For this review, take the finished solid that the model builds, in its own axes (mm). Face numbers are marked on the shaded views. A direction names the side the tool comes from. Coordinates: 2 decimals unless noted, no trailing zeros. Order: outer loops, then holes, each group sorted by start corner. A loop starts at its lowest first (then second) coordinate and runs counter-clockwise, first axis right, second up. Notation, with made-up numbers: (11.25, 24) -> (67.25, 24) arc R28 ccw to (67.25, 42) -> close; hole circle Ø1 at (5, 89.25). An arc over 180 degrees is marked (long way). Answer as a JSON object with one key per item and string values. Group by question number.
1) Add section C-C, the plane y = -20.5. Count the separate pieces of the cut face and the enclosed holes in it, then the cut area to 3 significant figures.
2) Add section B-B, the plane y = -36. Write out the cut boundary in (x, z).
3) Machinability: for the marked faces 1, 2, 3 and 4, which of the approach directions +Z, -Z, +X, -X, +Y, -Y give a long, thin tool a straight path to every point of the face, cutting with its end or side? Answer none if there is none.
4) For pin 1 (9 mm diameter, centred on y = -14, z = -31.5, fed in from -X); pin 2 (1 mm diameter, centred on y = -21, z = -8.5, fed in from +X); pin 3 (9 mm diameter, centred on y = -7.5, z = -28, fed in from +X); pin 4 (8 mm diameter, centred on x = 0.5, y = -35, fed in from +Z), all flat-tipped, find the tip position at first contact; note any pin that passes through.
5) Add section A-A, the plane z = 0. Write out the cut boundary in (x, y).
6) Add section D-D, the plane x = -16.5. Write out the cut boundary in (y, z), then the cut area to 3 significant figures.
7) Wall thickness on L1, parallel to X at y = -8, z = -29.5; L2, parallel to Z at x = 21.5, y = -3.5; L3, parallel to X at y = -27.5, z = -12.5: over which ranges is each line inside the solid? List them lowest first.
8) Draft analysis for pull direction X (two halves, no side actions). For the marked faces 5 and 6, state which applies: +X half, -X half, draft (parallel to the pull), parting line (faces both ways), or undercut.
from build123d import *

# Parameters (mm, degrees)
F0_W     = 86.6790302098
F0_H     = 110.9990477562
F0_R     = 4.1600175763
F0_R_2   = 4.0127427681
F1_DEPTH = 29.40571
F2_R     = 16.2901854198
F3_DEPTH = 25.4
F2_R_2   = 18.5490265687
F4_DEPTH = 30.0706941634
F6_R     = 15.7455659212
F7_DEPTH = 53.42441


with BuildPart() as f1:
    # F0 (on Front) → F1 (new body)
    with BuildSketch(Plane.XZ):
        with Locations((-5.9241037816, -20.7343772054)):
            Rectangle(F0_W, F0_H)
        with Locations((-28.4816268831, -32.2692543268)):
            Circle(F0_R, mode=Mode.SUBTRACT)
        with Locations((14.5424827933, -32.2692543268)):
            Circle(F0_R_2, mode=Mode.SUBTRACT)
        with BuildLine():
            add(Edge.make_bspline(
                [(-29.8793415714, -15.1079879142), (-29.0187247447, -16.080656118), (-29.0187247447, -17.7925521566)],
                knots=[0, 0, 0, 1, 1, 1], degree=2))
            add(Edge.make_bspline(
                [(-29.0187247447, -17.7925521566), (-29.0187247447, -19.4997793878), (-29.8824541096, -20.4778945335)],
                knots=[0, 0, 0, 1, 1, 1], degree=2))
            add(Edge.make_bspline(
                [(-29.8824541096, -20.4778945335), (-30.7461834745, -21.4560096792), (-32.2822211019, -21.4560096792)],
                knots=[0, 0, 0, 1, 1, 1], degree=2))
            add(Edge.make_bspline(
                [(-32.2822211019, -21.4560096792), (-33.8524966501, -21.4560096792), (-34.7061102657, -20.4950134939)],
                knots=[0, 0, 0, 1, 1, 1], degree=2))
            add(Edge.make_bspline(
                [(-34.7061102657, -20.4950134939), (-35.5597238813, -19.5340173086), (-35.5597238813, -17.7832145419)],
                knots=[0, 0, 0, 1, 1, 1], degree=2))
            add(Edge.make_bspline(
                [(-35.5597238813, -17.7832145419), (-35.5597238813, -16.0464181972), (-34.703775862, -15.0908689538)],
                knots=[0, 0, 0, 1, 1, 1], degree=2))
            add(Edge.make_bspline(
                [(-34.703775862, -15.0908689538), (-33.8478278427, -14.1353197105), (-32.2728834872, -14.1353197105)],
                knots=[0, 0, 0, 1, 1, 1], degree=2))
            add(Edge.make_bspline(
                [(-32.2728834872, -14.1353197105), (-30.739958398, -14.1353197105), (-29.8793415714, -15.1079879142)],
                knots=[0, 0, 0, 1, 1, 1], degree=2))
        make_face(mode=Mode.SUBTRACT)
        with BuildLine():
            Line((-23.1002332584, -21.3579647243), (-23.9079369348, -21.3579647243))
            Line((-23.9079369348, -21.3579647243), (-23.9079369348, -17.9092723411))
            add(Edge.make_bspline(
                [(-23.9079369348, -17.9092723411), (-23.9079369348, -17.2587518464), (-24.2044062034, -16.9373822719)],
                knots=[0, 0, 0, 1, 1, 1], degree=2))
            add(Edge.make_bspline(
                [(-24.2044062034, -16.9373822719), (-24.5008754719, -16.6160126973), (-25.1342770061, -16.6160126973)],
                knots=[0, 0, 0, 1, 1, 1], degree=2))
            add(Edge.make_bspline(
                [(-25.1342770061, -16.6160126973), (-25.9699935268, -16.6160126973), (-26.3590608083, -17.0681088784)],
                knots=[0, 0, 0, 1, 1, 1], degree=2))
            add(Edge.make_bspline(
                [(-26.3590608083, -17.0681088784), (-26.7481280898, -17.5202050596), (-26.7481280898, -18.5613491049)],
                knots=[0, 0, 0, 1, 1, 1], degree=2))
            Line((-26.7481280898, -18.5613491049), (-26.7481280898, -21.3579647243))
            Line((-26.7481280898, -21.3579647243), (-27.5558317662, -21.3579647243))
            Line((-27.5558317662, -21.3579647243), (-27.5558317662, -16.0277429677))
            Line((-27.5558317662, -16.0277429677), (-26.899086195, -16.0277429677))
            Line((-26.899086195, -16.0277429677), (-26.7683595885, -16.7576331878))
            Line((-26.7683595885, -16.7576331878), (-26.7294528603, -16.7576331878))
            add(Edge.make_bspline(
                [(-26.7294528603, -16.7576331878), (-26.4804498001, -16.3638970989), (-26.0330224264, -16.1467975558)],
                knots=[0, 0, 0, 1, 1, 1], degree=2))
            add(Edge.make_bspline(
                [(-26.0330224264, -16.1467975558), (-25.5855950527, -15.9296980128), (-25.0362320512, -15.9296980128)],
                knots=[0, 0, 0, 1, 1, 1], degree=2))
            add(Edge.make_bspline(
                [(-25.0362320512, -15.9296980128), (-24.0729014622, -15.9296980128), (-23.5865673603, -16.3942443469)],
                knots=[0, 0, 0, 1, 1, 1], degree=2))
            add(Edge.make_bspline(
                [(-23.5865673603, -16.3942443469), (-23.1002332584, -16.858790681), (-23.1002332584, -17.8812594968)],
                knots=[0, 0, 0, 1, 1, 1], degree=2))
            Line((-23.1002332584, -17.8812594968), (-23.1002332584, -21.3579647243))
        make_face(mode=Mode.SUBTRACT)
        with BuildLine():
            add(Edge.make_bspline(
                [(15.9240844259, -16.8496811724), (16.7484452225, -17.7813728502), (16.7484452225, -19.4211502033)],
                knots=[0, 0, 0, 1, 1, 1], degree=2))
            add(Edge.make_bspline(
                [(16.7484452225, -19.4211502033), (16.7484452225, -21.0564554363), (15.9211030126, -21.9933645876)],
                knots=[0, 0, 0, 1, 1, 1], degree=2))
            add(Edge.make_bspline(
                [(15.9211030126, -21.9933645876), (15.0937608026, -22.9302737389), (13.6224333049, -22.9302737389)],
                knots=[0, 0, 0, 1, 1, 1], degree=2))
            add(Edge.make_bspline(
                [(13.6224333049, -22.9302737389), (12.1183102601, -22.9302737389), (11.3006576436, -22.0097623611)],
                knots=[0, 0, 0, 1, 1, 1], degree=2))
            add(Edge.make_bspline(
                [(11.3006576436, -22.0097623611), (10.4830050271, -21.0892509834), (10.4830050271, -19.4122059632)],
                knots=[0, 0, 0, 1, 1, 1], degree=2))
            add(Edge.make_bspline(
                [(10.4830050271, -19.4122059632), (10.4830050271, -17.7485773032), (11.3028937036, -16.8332833988)],
                knots=[0, 0, 0, 1, 1, 1], degree=2))
            add(Edge.make_bspline(
                [(11.3028937036, -16.8332833988), (12.1227823802, -15.9179894945), (13.631377545, -15.9179894945)],
                knots=[0, 0, 0, 1, 1, 1], degree=2))
            add(Edge.make_bspline(
                [(13.631377545, -15.9179894945), (15.0997236293, -15.9179894945), (15.9240844259, -16.8496811724)],
                knots=[0, 0, 0, 1, 1, 1], degree=2))
        make_face(mode=Mode.SUBTRACT)
        with BuildLine():
            Line((20.4513606271, -17.730688823), (20.4513606271, -18.3314436169))
            Line((20.4513606271, -18.3314436169), (19.1514643981, -18.3314436169))
            Line((19.1514643981, -18.3314436169), (19.1514643981, -22.8363592178))
            Line((19.1514643981, -22.8363592178), (18.3777876288, -22.8363592178))
            Line((18.3777876288, -22.8363592178), (18.3777876288, -18.3314436169))
            Line((18.3777876288, -18.3314436169), (17.4654751378, -18.3314436169))
            Line((17.4654751378, -18.3314436169), (17.4654751378, -17.9826182527))
            Line((17.4654751378, -17.9826182527), (18.3777876288, -17.702365396))
            Line((18.3777876288, -17.702365396), (18.3777876288, -17.4191311259))
            add(Edge.make_bspline(
                [(18.3777876288, -17.4191311259), (18.3777876288, -15.5363685832), (20.0220371019, -15.5363685832)],
                knots=[0, 0, 0, 1, 1, 1], degree=2))
            add(Edge.make_bspline(
                [(20.0220371019, -15.5363685832), (20.4275093201, -15.5363685832), (20.9731079667, -15.6988556118)],
                knots=[0, 0, 0, 1, 1, 1], degree=2))
            Line((20.9731079667, -15.6988556118), (20.7718625643, -16.3189895926))
            add(Edge.make_bspline(
                [(20.7718625643, -16.3189895926), (20.3246505589, -16.1743910442), (20.0086207418, -16.1743910442)],
                knots=[0, 0, 0, 1, 1, 1], degree=2))
            add(Edge.make_bspline(
                [(20.0086207418, -16.1743910442), (19.5703529765, -16.1743910442), (19.3609086873, -16.4658242011)],
                knots=[0, 0, 0, 1, 1, 1], degree=2))
            add(Edge.make_bspline(
                [(19.3609086873, -16.4658242011), (19.1514643981, -16.7572573579), (19.1514643981, -17.399751939)],
                knots=[0, 0, 0, 1, 1, 1], degree=2))
            Line((19.1514643981, -17.399751939), (19.1514643981, -17.730688823))
            Line((19.1514643981, -17.730688823), (20.4513606271, -17.730688823))
        make_face(mode=Mode.SUBTRACT)
        with BuildLine():
            Line((23.684703426, -17.730688823), (23.684703426, -18.3314436169))
            Line((23.684703426, -18.3314436169), (22.384807197, -18.3314436169))
            Line((22.384807197, -18.3314436169), (22.384807197, -22.8363592178))
            Line((22.384807197, -22.8363592178), (21.6111304277, -22.8363592178))
            Line((21.6111304277, -22.8363592178), (21.6111304277, -18.3314436169))
            Line((21.6111304277, -18.3314436169), (20.6988179367, -18.3314436169))
            Line((20.6988179367, -18.3314436169), (20.6988179367, -17.9826182527))
            Line((20.6988179367, -17.9826182527), (21.6111304277, -17.702365396))
            Line((21.6111304277, -17.702365396), (21.6111304277, -17.4191311259))
            add(Edge.make_bspline(
                [(21.6111304277, -17.4191311259), (21.6111304277, -15.5363685832), (23.2553799009, -15.5363685832)],
                knots=[0, 0, 0, 1, 1, 1], degree=2))
            add(Edge.make_bspline(
                [(23.2553799009, -15.5363685832), (23.6608521191, -15.5363685832), (24.2064507656, -15.6988556118)],
                knots=[0, 0, 0, 1, 1, 1], degree=2))
            Line((24.2064507656, -15.6988556118), (24.0052053632, -16.3189895926))
            add(Edge.make_bspline(
                [(24.0052053632, -16.3189895926), (23.5579933578, -16.1743910442), (23.2419635407, -16.1743910442)],
                knots=[0, 0, 0, 1, 1, 1], degree=2))
            add(Edge.make_bspline(
                [(23.2419635407, -16.1743910442), (22.8036957754, -16.1743910442), (22.5942514862, -16.4658242011)],
                knots=[0, 0, 0, 1, 1, 1], degree=2))
            add(Edge.make_bspline(
                [(22.5942514862, -16.4658242011), (22.384807197, -16.7572573579), (22.384807197, -17.399751939)],
                knots=[0, 0, 0, 1, 1, 1], degree=2))
            Line((22.384807197, -17.399751939), (22.384807197, -17.730688823))
            Line((22.384807197, -17.730688823), (23.684703426, -17.730688823))
        make_face(mode=Mode.SUBTRACT)
    extrude(amount=F1_DEPTH)

    # F2 (on Front) → F3 (join)
    with BuildSketch(Plane.XZ):
        with Locations((-60.5162531137, 0)):
            Circle(F2_R)
    extrude(amount=F3_DEPTH)

    # F4 (add): a face of the model
    f4_faces = [f1.faces().sort_by_distance(p)[0] for p in [
        (-61.9656260946, -25.4, 0),
    ]]
    extrude(f4_faces, amount=F4_DEPTH)

    # F6 (on Front) → F7 (join)
    with BuildSketch(Plane.XZ):
        with Locations((49.0159541368, 0)):
            Circle(F6_R)
    extrude(amount=F7_DEPTH)


with BuildPart() as f3:
    # F2 (on Front) → F3, piece 2 (new body)
    with BuildSketch(Plane.XZ):
        with Locations((56.2986545265, 0)):
            Circle(F2_R_2)
    extrude(amount=F3_DEPTH)


solid = f1.part
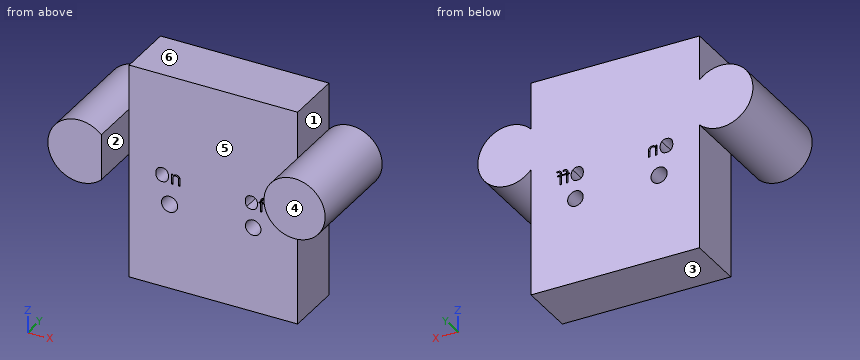
Output values:
{
 "1": {"separate pieces": "1", "enclosed holes": "7", "area": "10,900 mm²"},
 "2": {"outline": "(-49.26, -11.78) -> (-49.26, 11.78) arc R16.29 ccw (long way) to start; circle Ø31.49 at (49.02, 0)"},
 "3": {"face 1": "+Z, +Y, -Y", "face 2": "+Z, -Z, -Y", "face 3": "-Z, +X, -X, +Y, -Y", "face 4": "+Z, -Z, +X, -Y"},
 "4": {"pin 1": "stops at x = -49.26", "pin 2": "stops at x = 62.58", "pin 3": "stops at x = 37.42", "pin 4": "passes through"},
 "5": {"outline": "(-76.81, -55.47) -> (-49.26, -55.47) -> (-49.26, -29.41) -> (33.27, -29.41) -> (33.27, -53.42) -> (64.76, -53.42) -> (64.76, 0) -> (-76.81, 0) -> close"},
 "6": {"outline": "(-29.41, -76.23) -> (0, -76.23) -> (0, 34.77) -> (-29.41, 34.77) -> close", "area": "3,260 mm²"},
 "7": {"L1": "x = -49.26 to -31.59, -25.38 to 11.64, 17.45 to 37.42", "L2": "z = -76.23 to -18.33, -17.74 to 34.77", "L3": "x = -70.96 to -50.07, -49.26 to 37.42, 39.44 to 58.59"},
 "8": {"face 5": "undercut", "face 6": "draft"}
}
